Verification items for the finished model (mm, model axes). Coordinates: 2 decimals unless noted, no trailing zeros. Write each loop counter-clockwise with the first axis right and the second up, starting at its lowest first coordinate (ties: lowest second). Pieces come first, ordered by that corner, then holes. Notation, with made-up numbers: (-21, 40.25) -> (25, 40.25) arc R7 ccw to (25, 47.25) -> close; hole circle Ø3 at (69, 14.5). An arc over 180 degrees is marked (long way). Answer in a Markdown table with one row per item.
```python
from build123d import *

# Parameters (mm, degrees)
SKETCH1_W                                      = 180.975
SKETCH1_H                                      = 133.35
SKETCH1_W_2                                    = 165.408
SKETCH1_H_2                                    = 102.508
BOSS_EXTRUDE1_DEPTH                            = 5.842
FILLET2_R                                      = 12.7
CBORE_FOR_M3_SHCS1_D                           = 3.4
CBORE_FOR_M3_SHCS1_DEPTH                       = 4.064
CBORE_FOR_M3_SHCS1_CBORE_D                     = 6.5
CBORE_FOR_M3_SHCS1_CBORE_DEPTH                 = 3
CBORE_FOR_M3_SHCS1_TIP                         = 1.021463052
CBORE_FOR_M3_SHCS2_D                           = 3.6
CBORE_FOR_M3_SHCS2_DEPTH                       = 5.842
CBORE_FOR_M3_SHCS2_CBORE_D                     = 6.5
CBORE_FOR_M3_SHCS2_CBORE_DEPTH                 = 3
MIRROR1_AT_THE_SECOND_PLANE_COPY_1_D           = 3.6
MIRROR1_AT_THE_SECOND_PLANE_COPY_1_DEPTH       = 5.842
MIRROR1_AT_THE_SECOND_PLANE_COPY_1_CBORE_D     = 6.5
MIRROR1_AT_THE_SECOND_PLANE_COPY_1_CBORE_DEPTH = 3


with BuildPart() as part:
    # Sketch1 → Boss-Extrude1 (new body)
    with BuildSketch(Plane.XY):
        with Locations((78.461, -0.01)):
            Rectangle(SKETCH1_W, SKETCH1_H)
        with Locations((78.461, -0.01)):
            Rectangle(SKETCH1_W_2, SKETCH1_H_2, mode=Mode.SUBTRACT)
    extrude(amount=BOSS_EXTRUDE1_DEPTH)

    # Fillet2
    fillet2_edges = [part.edges().sort_by_distance(p)[0] for p in [
        (168.9485, -66.685, 2.921),
        (168.9485, 66.665, 2.921),
        (-12.0265, 66.665, 2.921),
        (-12.0265, -66.685, 2.921),
    ]]
    fillet(fillet2_edges, radius=FILLET2_R)

    # CBORE for M3 SHCS1
    with Locations(Plane.XY.offset(5.842)):
        with Locations((0, 57.785), (156.922, 57.785), (156.922, -57.785), (0, -57.785)):
            CounterBoreHole(CBORE_FOR_M3_SHCS1_D / 2, CBORE_FOR_M3_SHCS1_CBORE_D / 2, CBORE_FOR_M3_SHCS1_CBORE_DEPTH, depth=CBORE_FOR_M3_SHCS1_DEPTH)
            with Locations((0, 0, -(CBORE_FOR_M3_SHCS1_DEPTH + CBORE_FOR_M3_SHCS1_TIP / 2))):  # 118° drill point
                Cone(0, CBORE_FOR_M3_SHCS1_D / 2, CBORE_FOR_M3_SHCS1_TIP, mode=Mode.SUBTRACT)

    # CBORE for M3 SHCS2
    with Locations(Plane.XY.offset(5.842)):
        with Locations((38.1, 57.785), (-8.306756121, 32.385)):
            cbore_for_m3_shcs2 = CounterBoreHole(CBORE_FOR_M3_SHCS2_D / 2, CBORE_FOR_M3_SHCS2_CBORE_D / 2, CBORE_FOR_M3_SHCS2_CBORE_DEPTH, depth=CBORE_FOR_M3_SHCS2_DEPTH)

    # Mirror1: CBORE for M3 SHCS2 across plane
    add(cbore_for_m3_shcs2.mirror(Plane(origin=(0, -0.01, 0), x_dir=(0, 0, 1), z_dir=(0, -1, 0))), mode=Mode.SUBTRACT)

    # Mirror1 at the second plane: CBORE for M3 SHCS2 across plane
    add(cbore_for_m3_shcs2.mirror(Plane(origin=(78.461, 0, 0), x_dir=(0, 0, 1), z_dir=(1, 0, 0))), mode=Mode.SUBTRACT)

    # Mirror1 at the second plane copy 1
    with Locations(Plane(origin=(156.922, -0.02, 5.842), x_dir=(-1, 0, 0), z_dir=(0, 0, 1))):
        with Locations((38.1, 57.785), (-8.306756121, 32.385)):
            CounterBoreHole(MIRROR1_AT_THE_SECOND_PLANE_COPY_1_D / 2, MIRROR1_AT_THE_SECOND_PLANE_COPY_1_CBORE_D / 2, MIRROR1_AT_THE_SECOND_PLANE_COPY_1_CBORE_DEPTH, depth=MIRROR1_AT_THE_SECOND_PLANE_COPY_1_DEPTH)


solid = part.part
```
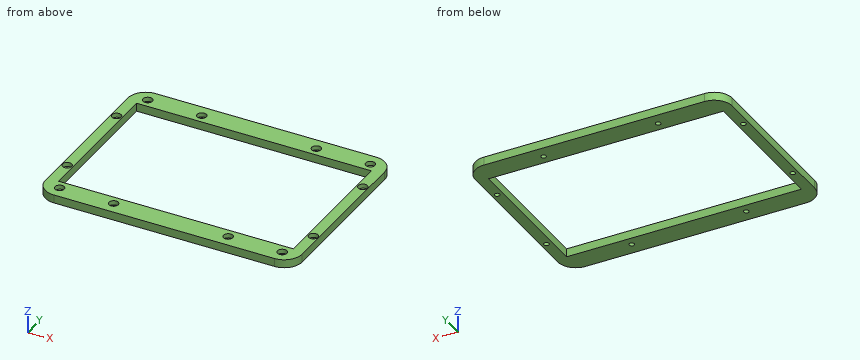
1. Sectioned sample at A-A, the plane x = 20.5. Record the cut outline in (y, z) (3 decimals).
Findings below:
| item | result |
|---|---|
| outline | (-66.685, 0) -> (-51.264, 0) -> (-51.264, 5.842) -> (-66.685, 5.842) -> close; (51.244, 0) -> (66.665, 0) -> (66.665, 5.842) -> (51.244, 5.842) -> close |
2. Sectioned sample at B-B, the plane y = -43. Record the cut outline in (x, z) (1 decimal).
Findings below:
| item | result |
|---|---|
| outline | (-12, 0) -> (-4.2, 0) -> (-4.2, 5.8) -> (-12, 5.8) -> close; (161.2, 0) -> (168.9, 0) -> (168.9, 5.8) -> (161.2, 5.8) -> close |
3. Go/stop test with flat-tipped pins: pin 1 (2 mm diameter, centred on x = 118.5, y = 59, fed in from +Z); pin 2 (2.5 mm diameter, centred on x = 0, y = 57.785, fed in from +Z). Record where each tip stops, or that it passes through.
Findings below:
| item | result |
|---|---|
| pin 1 | stops at z = 2.84 |
| pin 2 | stops at z = 1.51 |
4. Material ranges on probe 1 along Y at (x, z) = (110, 2.7) (3 decimals); probe 2 along X at (y, z) = (32, 3.1) (1 decimal); probe 3 along X at (y, z) = (-17.5, 0.85) (1 decimal), recorded low to high. Write a range as from..to.
Findings below:
| item | result |
|---|---|
| probe 1 | y = -66.685..-51.264, 51.244..66.665 |
| probe 2 | x = -12..-11.5, -5.1..-4.2, 161.2..162, 168.5..168.9 |
| probe 3 | x = -12..-4.2, 161.2..168.9 |
